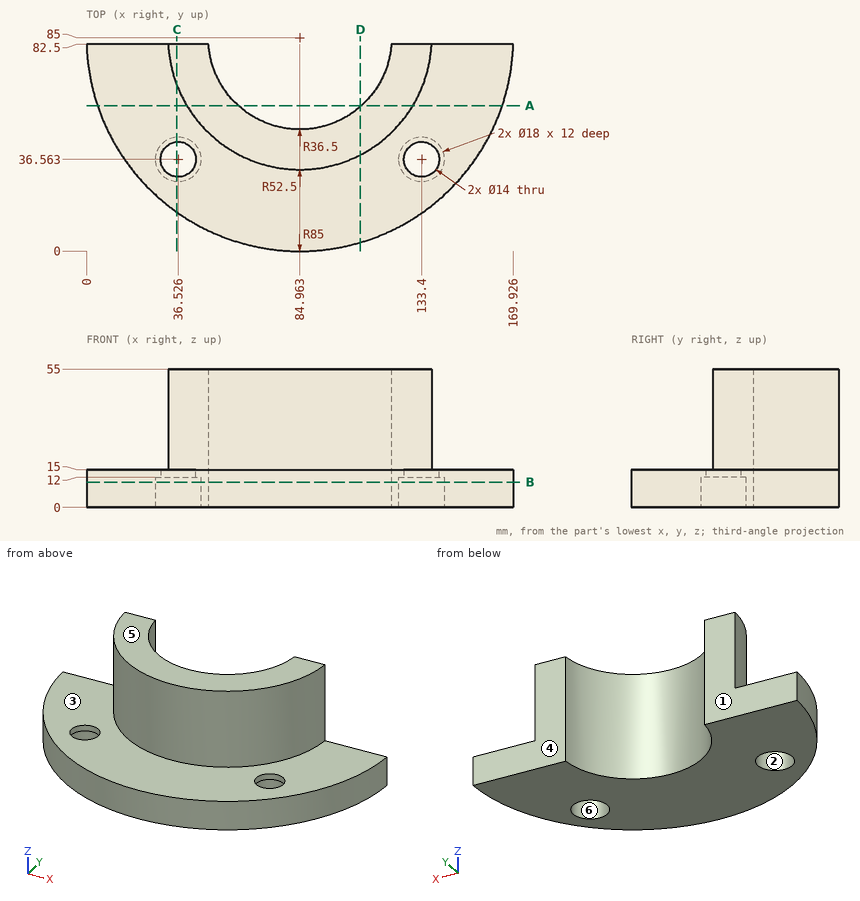
Answer from the drawing. Dimensions are ordinates in mm from the lowest x, y and z of the part. A direction names the side the tool comes from. Coordinates: 2 decimals unless noted, no trailing zeros. Loops run counter-clockwise (first coordinate to the right, second up) from the corner with the lowest first, then second, coordinate; pieces in that order, holes last. Notation, with made-up numbers: (32.25, -40) -> (68.25, -40) arc R20 cw to (68.25, -17) -> close; hole circle Ø8 at (25.5, -36.75). An arc over 180 degrees is marked (long way). Answer as CSV lines item,"result".
Q1. A tool of negligible diameter and unlimited length cuts with its end or side. For the marked faces 1, 2 and 3, from which of +Z, -Z, +X, -X, +Y, -Y can it reach the whole face along a straight path? Write none if from no direction.
Findings:
face 1,"+Z, -Z, +X, -X, +Y"
face 2,"-Z"
face 3,"+Z, -Y"
Q2. The part is cut by section C-C on x = 36. Write down the section's boundary in (y, z), and give its area (4 significant figures).
Findings:
outline,"(15.52, 0) -> (27.58, 0) -> (27.58, 12) -> (29.58, 12) -> (29.58, 15) -> (15.52, 15) -> close; (43.54, 12) -> (45.55, 12) -> (45.55, 0) -> (82.5, 0) -> (82.5, 55) -> (66.06, 55) -> (66.06, 15) -> (43.54, 15) -> close"
area,"1,405 mm²"
Q3. Find the intervals of material crossed by probe 1 along X at (y, z) = (38.5, 8.5) (1 decimal); probe 2 along X at (y, z) = (32, 6) (1 decimal); probe 3 along Z at (x, y) = (67.5, 35), in increasing order.
Findings:
probe 1,"x = 13.8 to 27.7, 45.3 to 124.6, 142.2 to 156.1"
probe 2,"x = 18.5 to 28.8, 44.3 to 125.6, 141.2 to 151.4"
probe 3,"z = 0 to 15"
Q4. The part is cut by section B-B on z = 10. Write down the section's boundary in (x, y).
Findings:
outline,"(0, 82.5) arc R85 ccw to (169.93, 82.5) -> (121.38, 82.5) arc R36.5 cw to (48.55, 82.5) -> close; hole circle Ø18 at (36.53, 36.56); hole circle Ø18 at (133.4, 36.56)"
Q5. For a pull along Y with two mould halves and no side action, classify the marked faces 4, 5 and 6 as +Y half, -Y half, draft (parallel to the pull), parting line (faces both ways), or undercut.
Findings:
face 4,"+Y half"
face 5,"draft"
face 6,"undercut"
Q6. The part is cut by section D-D on x = 109. Write down the section's boundary in (y, z) (1 decimal).
Findings:
outline,"(3.5, 0) -> (57.5, 0) -> (57.5, 55) -> (38.3, 55) -> (38.3, 15) -> (3.5, 15) -> close"
Q7. Each of these flat-tipped pins is pushed along its axis until it touches: pin 1 (2 mm diameter, centred on y = 70, z = 19.5, fed in from +X); pin 2 (4 mm diameter, centred on y = 40, z = 44, fed in from +X) (1 decimal); pin 3 (22.5 mm diameter, centred on x = 133.4, y = 36.56, fed in from +Z). Where does it stop, or does it pass through?
Findings:
pin 1,"stops at x = 135.56"
pin 2,"stops at x = 115.1"
pin 3,"stops at z = 15"
Q8. The part is cut by section A-A on y = 58. Write down the section's boundary in (x, z) (1 decimal).
Findings:
outline,"(4.4, 0) -> (60.4, 0) -> (60.4, 55) -> (39.9, 55) -> (39.9, 15) -> (4.4, 15) -> close; (109.5, 0) -> (165.6, 0) -> (165.6, 15) -> (130, 15) -> (130, 55) -> (109.5, 55) -> close"
